Input: part model. Units: mm. Frame: model coordinates. Face numbers are marked on the shaded views. A direction names the side the tool comes from. Coordinates: 2 decimals unless noted, no trailing zeros. Loops run counter-clockwise (first coordinate to the right, second up) from the corner with the lowest first, then second, coordinate; pieces in that order, holes last.
(1) Section D-D, the plane z = 1.5. Return loops of the section in (x, y).
(2) Contact query for flat-ended pins moving along their axis: P1, Ø21, axis at x = 28.5, y = -11, coming from the -Z side; P2, Ø2, axis at x = 66.5, y = 14.5, coming from the -Z side; P3, Ø2, axis at x = 4.5, z = -5, coming from the +Y side; P4, Ø6.5, axis at x = 22.45, y = -51.53, coming from the +Z side. Output: stop coordinate, or through.
(3) Mould query, pull axis X, two halves, no side actions, for the marked faces 1, 2 and 3. Classes: released by +X, released by -X, zero draft, split by the parting line, or undercut.
(4) Section C-C, the plane x = 75. Return loops of the section in (y, z), then the cut area to 3 significant figures.
(5) Set-up query: the marked faces 4, 5 and 6. Return all of +Z, -Z, +X, -X, +Y, -Y with unobstructed straight access to the full face (end or side cutting, diameter ignored); none if empty.
(6) Line query: L1, parallel to Z at x = 56, y = -21.5; L2, parallel to X at y = -52, z = 10.5; L3, parallel to Z at x = 32, y = 52. Output: solid intervals per line, ascending.
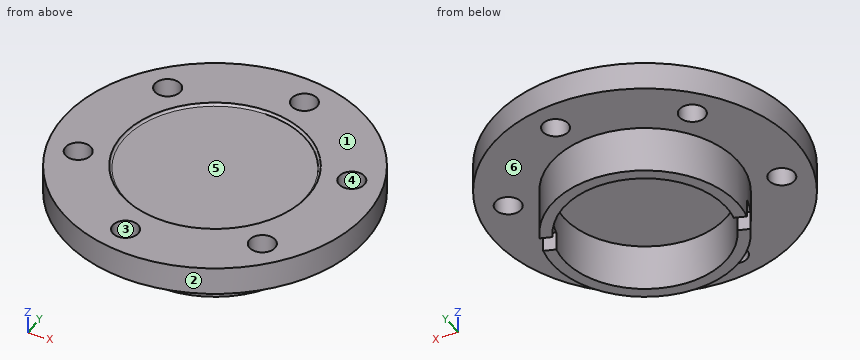
Autodesk Inventor part; units mm, degrees
ref_plane "工作平面1" through (0, 0, 0) normal (0, 0, 1) x (1, 0, 0)
ref_plane "工作平面2" through (-0.3829, -11.3012, -12) normal (-0.325, 0.9457, 0) x (0.9457, 0.325, 0)
ref_plane "YZ Plane" through (0, 0, 0) normal (1, 0, 0) x (0, 1, 0)
ref_plane "工作平面1" through (0, 0, 0) normal (0, 0, 1) x (1, 0, 0)
sketch "草图1" plane through (0, 0, 0) normal (0, 0, 1) x (1, 0, 0)
  arc A0 (32.5, 65) -> (32.5, -65) centre (32.5, 0) ccw construction
  line L0 (32.5, -65) -> (32.5, -40) construction
  arc A1 (32.5, 40) -> (32.5, -40) centre (32.5, 0) ccw construction
  line L1 (32.5, 40) -> (32.5, 65) construction
  circle A2 centre (32.5, 0) radius 65
  circle A3 centre (72.1024, -34.466) radius 5.5
  circle A4 centre (-17.1496, -17.0637) radius 5.5
  circle A5 centre (82.1496, 17.0637) radius 5.5
  circle A6 centre (42.5472, 51.5296) radius 5.5
  circle A7 centre (22.4528, -51.5296) radius 5.5
  circle A8 centre (-7.1024, 34.466) radius 5.5
  circle A9 centre (32.5, 0) radius 65
  circle A10 centre (32.5, 0) radius 40 construction
  point P0 (0, 0)
extrude "拉伸1" add sketch "草图1" along normal blind 12
sketch "草图2" plane through (32.5, 0, 0) normal (0, 0, -1) x (-1, 0, 0)
  circle A0 centre (0, 0) radius 65 construction
  circle A1 centre (0, 0) radius 40
  circle A2 centre (0, 0) radius 35
  point P0 (32.5, 0)
  dimension "d2" = 80
  dimension "d3" = 70
extrude "拉伸2" add sketch "草图2" along normal blind 20
sketch "草图3" plane through (32.5, 0, 12) normal (0, 0, 1) x (1, 0, 0)
  circle A0 centre (0, 0) radius 65 construction
  circle A1 centre (0, 0) radius 40
  point P0 (-32.5, 0)
  dimension "d6" = 80
extrude "拉伸3" cut sketch "草图3" against normal blind 1
fillet "圆角1" radius 1 1 edges at (-7.5, 0, 11)
sketch "草图4" plane through (32.5, 0, -20) normal (0, 0, -1) x (-1, 0, 0)
  circle A0 centre (0, 0) radius 35 construction
  circle A1 centre (49.6496, -17.0637) radius 5.5 construction
  circle A2 centre (-49.6496, 17.0637) radius 5.5 construction
  line L0 (49.6496, -17.0637) -> (-49.6496, 17.0637) construction
  line L1 (66.9706, -27.2462) -> (-94.2998, 28.1795)
  line L2 (-94.2998, 28.1795) -> (-91.6996, 35.7451)
  line L3 (-91.6996, 35.7451) -> (69.5708, -19.6806)
  line L4 (69.5708, -19.6806) -> (66.9706, -27.2462)
  point P0 (32.5, 0)
  dimension "d10" = 8
extrude "拉伸4" cut sketch "草图4" against normal blind 8
ref_plane "工作平面2" through (-0.3829, -11.3012, -12) normal (-0.325, 0.9457, 0) x (0.9457, 0.325, 0)
properties part number "轴承通盖1"
Report:
1. outline: circle Ø130 at (32.5, 0); hole circle Ø11 at (-17.15, -17.06); hole circle Ø11 at (-7.1, 34.47); hole circle Ø11 at (22.45, -51.53); hole circle Ø11 at (42.55, 51.53); hole circle Ø11 at (72.1, -34.47); hole circle Ø11 at (82.15, 17.06)
2. P1: stops at z = 0
2. P2: stops at z = -12
2. P3: stops at y = 29.51
2. P4: passes through
3. face 1: zero draft
3. face 2: split by the parting line
3. face 3: undercut
4. outline: (-49.18, 0) - (-39.14, 0) - (-39.14, 12) - (-49.18, 12) - close; (-29.79, 0) - (49.18, 0) - (49.18, 12) - (-29.79, 12) - close
4. area: 1,070 mm2
5. face 4: +Z, -Z
5. face 5: +Z
5. face 6: -Z
6. L1: z = 0 to 11
6. L2: x = -6.5 to 16.97, 27.93 to 71.5
6. L3: z = 0 to 12
